```python
from build123d import *

# Parameters (mm, degrees)
SKETCH_1_R          = 38.25
EXTRUDE_1_DEPTH     = 5
FILLET_1_R          = 5
SKETCH_5_R          = 8
CUT_EXTRUDE_1_DEPTH = 66.0000001
SKETCH_6_W          = 20
SKETCH_6_H          = 20
EXTRUDE_2_DEPTH     = 10


with BuildPart() as part:
    # ｽｹｯﾁ1 → ﾎﾞｽ - 押し出し1 (new body)
    with BuildSketch(Plane.XY):
        Circle(SKETCH_1_R)
    extrude(amount=EXTRUDE_1_DEPTH)

    # ｽｹｯﾁ2 → 回転1 (revolve)
    with BuildSketch(Plane(origin=(0, 0, 0), x_dir=(0, 0, -1), z_dir=(1, 0, 0))):
        Polygon((-22, 0), (-22, 15), (-9, 17), (-5, 38.25), (-5, 0), align=None)
    revolve(axis=Axis((0, 0, 0), (0, 0, 1)))

    # ﾌｨﾚｯﾄ1
    fillet_1_edges = [part.edges().sort_by_distance(p)[0] for p in [
        (0, -17, 9),
    ]]
    fillet(fillet_1_edges, radius=FILLET_1_R)

    # ｽｹｯﾁ3 → 回転2 (revolve)
    with BuildSketch(Plane(origin=(0, 0, 0), x_dir=(0, 0, -1), z_dir=(1, 0, 0))):
        with BuildLine():
            Line((-45, 26.1), (-33, 26.1))
            add(Edge.make_bspline(
                [(-33, 26.1), (-30.010138273, 26.1), (-26.820768311, 24.254113599), (-25.622496591, 23.557974687), (-22.470712298, 20.950193944), (-22, 15)],
                knots=[0, 0, 0, 0, 0.463324442, 0.563324442, 1, 1, 1, 1], degree=3))
            Line((-22, 15), (-22, 0))
            Line((-22, 0), (-57.35662508, 0))
            Line((-57.35662508, 0), (-65, 21))
            add(Edge.make_bspline(
                [(-45, 26.1), (-57.846202283, 26.003969711), (-64.230299253, 22.294062624), (-65, 21)],
                knots=[0, 0, 0, 0, 1, 1, 1, 1], degree=3))
        make_face()
    revolve(axis=Axis((0, 0, 0), (0, 0, 1)))

    # ｽｹｯﾁ5 → ｶｯﾄ - 押し出し1 (cut, through all)
    with BuildSketch(Plane(origin=(0, 0, 0), x_dir=(-1, 0, 0), z_dir=(0, 0, -1))):
        Circle(SKETCH_5_R)
    extrude(amount=-CUT_EXTRUDE_1_DEPTH, mode=Mode.SUBTRACT)

    # ｽｹｯﾁ6 → ﾎﾞｽ - 押し出し2 (add)
    with BuildSketch(Plane(origin=(0, 0, 0), x_dir=(-1, 0, 0), z_dir=(0, 0, -1))):
        Rectangle(SKETCH_6_W, SKETCH_6_H)
    extrude(amount=EXTRUDE_2_DEPTH)


solid = part.part
```
The model under review builds one solid part; all positions refer to its coordinate system, in mm. A direction names the side the tool comes from. Round coordinates to 2 decimals unless told otherwise and drop trailing zeros. Order: outer loops, then holes, each group sorted by start corner. A loop starts at its lowest first (then second) coordinate and runs counter-clockwise, first axis right, second up. Notation, with made-up numbers: (78.5, 16.5) -> (100.5, 16.5) arc R14 cw to (100.5, 39.5) -> close; hole circle Ø7 at (-39, 43.25). An arc over 180 degrees is marked (long way). One line per item, written item: value. Start each with the question number.
Q1. Mouldability with a two-part tool opening along Y and no side actions: class faces 4 (the face through (8.604, -1.911, 60.564)), 5 (the face through (10, 0, -5)), 6 (the face through (0, 10, -5)) as released by +Y, released by -Y, zero draft, split by the parting line, or undercut.
Q2. Take a section at B-B (z = 14.5). Write out the cut boundary in (x, y).
Q3. Clearance check with flat-ended pins moving along their axes: pin 1 Ø11 at (x, z) = (5, -6) entering from +Y; pin 2 Ø3 at (x, z) = (-21, 48) entering from -Y; pin 3 Ø8 at (y, z) = (4.5, -5.5) entering from -X; pin 4 Ø23 at (x, y) = (1.5, -12) entering from -Z. State where each tip first meets the part, or that it passes through.
Q4. Wall thickness on line 1 (X direction, y = 0, z = 45.5); line 2 (Y direction, x = 0, z = 33); line 3 (X direction, y = 0, z = 47): over which ranges is each line inside the solid? List them lowest first.
Q5. Take a section at A-A (z = -5). Write out the cut boundary in (x, y), and give its area (3 significant figures).
Q6. Machinability: for faces 1 (the face through (-10, 0, -5)), 2 (the face through (0, -10, -5)), 3 (the face through (1.73, -7.81, 29.71)), which of the approach directions +Z, -Z, +X, -X, +Y, -Y give a long, thin tool a straight path to every point of the face, cutting with its end or side? Answer none if there is none.
Reported:
1. face 4: undercut
1. face 5: zero draft
1. face 6: released by +Y
2. outline: circle Ø32.31 at (0, 0); hole circle Ø16 at (0, 0)
3. pin 1: stops at y = 10
3. pin 2: stops at y = -17.21
3. pin 3: stops at x = -10
3. pin 4: stops at z = -10
4. line 1: x = -26.09 to -8, 8 to 26.09
4. line 2: y = -26.1 to -8, 8 to 26.1
4. line 3: x = -26.05 to -8, 8 to 26.05
5. outline: (-10, -10) -> (10, -10) -> (10, 10) -> (-10, 10) -> close
5. area: 400 mm2
6. face 1: -Z, -X, +Y, -Y
6. face 2: -Z, +X, -X, -Y
6. face 3: +Z
